The model under review builds one solid part; all positions refer to its coordinate system, in mm. Face numbers are marked on the shaded views. A direction names the side the tool comes from. Give positions to 0.01 mm unless a question says otherwise; leave off trailing zeros. Write each loop counter-clockwise with the first axis right and the second up, starting at its lowest first coordinate (ties: lowest second). Pieces come first, ordered by that corner, then holes.
from build123d import *

# Parameters (mm, degrees)
Y_KSEKLIK_EKSTR_ZYON1_DEPTH = 38.1
KES_EKSTR_ZYON1_REACH       = 142.901
IZIM2_R                     = 6.35
KES_EKSTR_ZYON2_REACH       = 151.446
IZIM3_R                     = 4.765


with BuildPart() as part:
    # Çizim1 → Yükseklik-Ekstrüzyon1 (new body)
    with BuildSketch(Plane(origin=(0, 0, 0), x_dir=(0, 0, -1), z_dir=(1, 0, 0))):
        with BuildLine():
            Line((0, 0), (63.51, 0))
            ThreePointArc((63.51, 0), (70.248727625, -2.791272375), (73.04, -9.53))
            Line((73.04, -9.53), (73.04, -104.78))
            ThreePointArc((73.04, -104.78), (70.248727625, -111.518727625), (63.51, -114.31))
            Line((63.51, -114.31), (9.39, -114.31))
            ThreePointArc((9.39, -114.31), (5.332325351, -113.403002751), (2.047011614, -110.854654028))
            Line((2.047011614, -110.854654028), (-26.694452199, -76.112225243))
            Line((-26.694452199, -76.112225243), (-21.801694985, -72.064580639))
            Line((-21.801694985, -72.064580639), (6.939768828, -106.807009424))
            ThreePointArc((6.939768828, -106.807009424), (8.03602252, -107.657350341), (9.39, -107.96))
            Line((9.39, -107.96), (63.51, -107.96))
            ThreePointArc((63.51, -107.96), (65.758599564, -107.028599564), (66.69, -104.78))
            Line((66.69, -104.78), (66.69, -9.53))
            ThreePointArc((66.69, -9.53), (65.758599564, -7.281400436), (63.51, -6.35))
            Line((63.51, -6.35), (0, -6.35))
            Line((0, -6.35), (0, 0))
        make_face()
    extrude(amount=Y_KSEKLIK_EKSTR_ZYON1_DEPTH)

    # Çizim2 → Kes-Ekstrüzyon1 (cut, up to next)
    with BuildSketch(Plane(origin=(0, 0, 0), x_dir=(1, 0, 0), z_dir=(0, 1, 0)), mode=Mode.PRIVATE) as kes_ekstr_zyon1_sk1:
        with Locations(Location((19.05, 19.04, 0), (0, 0, 270))):
            Circle(IZIM2_R)
    kes_ekstr_zyon1_tool1 = extrude(kes_ekstr_zyon1_sk1.sketch, amount=-KES_EKSTR_ZYON1_REACH, mode=Mode.PRIVATE) & part.part
    add(kes_ekstr_zyon1_tool1.solids().sort_by_distance((19.05, 0, -19.04))[0], mode=Mode.SUBTRACT)

    # Çizim3 → Kes-Ekstrüzyon2 (cut, up to next)
    with BuildSketch(Plane(origin=(0, -44.03595524, 53.230275565), x_dir=(1, 0, 0), z_dir=(0, -0.6374243471515584, 0.770512947106283)), mode=Mode.PRIVATE) as kes_ekstr_zyon2_sk1:
        with Locations(Location((19.05, -62.439761218, 0), (0, 0, 270))):
            Circle(IZIM3_R)
    kes_ekstr_zyon2_tool1 = extrude(kes_ekstr_zyon2_sk1.sketch, amount=-KES_EKSTR_ZYON2_REACH, mode=Mode.PRIVATE) & part.part
    add(kes_ekstr_zyon2_tool1.solids().sort_by_distance((19.05, -92.1466, 13.429652))[0], mode=Mode.SUBTRACT)


solid = part.part
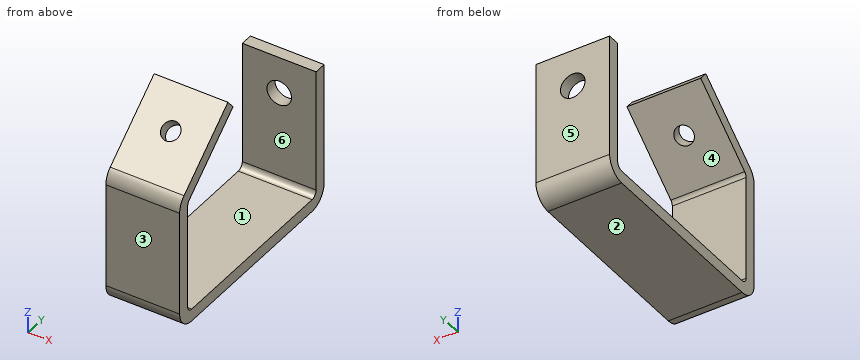
1) Consider section C-C, the plane x = 19.05. Give the boundary of the cut face in (y, z), then the cut area to 3 significant figures.
2) To check wall thickness, follow probe 1 along Y at (x, z) = (23, -48); probe 2 along X at (y, z) = (-3, -19); probe 3 along Y at (x, z) = (14.5, -19.5). State the ranges of each line that lie inside material, in increasing order.
3) Consider section B-B, the plane z = -32.5. Give the boundary of the cut face in (x, y), then the cut area to 3 significant figures.
4) Insertion check: pin 1 (11.5 mm diameter, centred on x = 16, y = -73, fed in from +Z); pin 2 (4 mm diameter, centred on y = -82, z = 8.5, fed in from -X); pin 3 (14.5 mm diameter, centred on x = 19.05, z = -19.04, fed in from +Y); pin 4 (4 mm diameter, centred on x = 19, y = -86, fed in from +Z). Each pin has a flat end and moves straight along its axis. Give the tip position at first contact, or say it passes through.
5) Consider section A-A, the plane z = -19.04. Give the boundary of the cut face in (x, y).
6) Consider section D-D, the plane y = -73.5. Give the boundary of the cut face in (x, z).
7) Tool access review of the marked faces 4, 5 and 6: name each direction out of +Z, -Z, +X, -X, +Y, -Y from which nothing blocks a thin tool from reaching the whole face with its end or side.
8) The part is to be moulded in two halves that separate along Y. For the marked faces 1, 2 and 3, say which applies: +Y half, -Y half, draft (parallel to the pull), parting line (faces both ways), or undercut.
Answer block:
1. outline: (-114.31, -63.51) arc R9.53 ccw to (-104.78, -73.04) - (-9.53, -73.04) arc R9.53 ccw to (0, -63.51) - (0, -25.39) - (-6.35, -25.39) - (-6.35, -63.51) arc R3.18 cw to (-9.53, -66.69) - (-104.78, -66.69) arc R3.18 cw to (-107.96, -63.51) - (-107.96, -9.39) arc R3.18 cw to (-106.81, -6.94) - (-91.77, 5.5) - (-95.82, 10.39) - (-110.85, -2.05) arc R9.53 ccw to (-114.31, -9.39) - close; (-88.48, 16.47) - (-84.43, 11.57) - (-72.06, 21.8) - (-76.11, 26.69) - close; (-6.35, -12.69) - (0, -12.69) - (0, 0) - (-6.35, 0) - close
1. area: 1,660 mm2
2. probe 1: y = -114.31 to -107.96, -6.35 to 0
2. probe 2: x = 0 to 12.7, 25.4 to 38.1
2. probe 3: y = -114.31 to -107.96
3. outline: (0, -114.31) - (38.1, -114.31) - (38.1, -107.96) - (0, -107.96) - close; (0, -6.35) - (38.1, -6.35) - (38.1, 0) - (0, 0) - close
3. area: 484 mm2
4. pin 1: stops at z = 26.69
4. pin 2: passes through
4. pin 3: stops at y = 0
4. pin 4: stops at z = 20.17
5. outline: (0, -114.31) - (38.1, -114.31) - (38.1, -107.96) - (0, -107.96) - close; (0, -6.35) - (12.7, -6.35) - (12.7, 0) - (0, 0) - close; (25.4, -6.35) - (38.1, -6.35) - (38.1, 0) - (25.4, 0) - close
6. outline: (0, -73.04) - (38.1, -73.04) - (38.1, -66.69) - (0, -66.69) - close; (0, 20.61) - (38.1, 20.61) - (38.1, 23.54) - (0, 23.54) - close
7. face 4: +X, -X
7. face 5: +Z, -Z, +X, -X, +Y
7. face 6: +Z, +X, -X
8. face 1: undercut
8. face 2: draft
8. face 3: -Y half
